from build123d import *

# Parameters (mm, degrees)
FILLET2_R = 2.1


with BuildPart() as part:
    # Sketch1 → Revolve1 (revolve)
    with BuildSketch(Plane(origin=(0, 0, 0), x_dir=(1, 0, 0), z_dir=(0, 1, 0)), mode=Mode.PRIVATE) as revolve1_sk:
        with BuildLine():
            Line((152.17858106, 53), (144.228415495, 53))
            ThreePointArc((144.228415495, 53), (136.67858106, 56), (129.128746624, 53))
            Line((129.128746624, 53), (121.17858106, 53))
            Line((121.17858106, 53), (121.17858106, 65))
            Line((121.17858106, 65), (152.17858106, 65))
            Line((152.17858106, 65), (152.17858106, 53))
        make_face()
    revolve(revolve1_sk.sketch.rotate(Axis((-165.426008969, 0, 0), (1, 0, 0)), 180), axis=Axis((-165.426008969, 0, 0), (1, 0, 0)))

    # Fillet2
    fillet2_edges = [part.edges().sort_by_distance(p)[0] for p in [
        (152.17858106, 0, -65),
        (121.17858106, 0, -65),
    ]]
    fillet(fillet2_edges, radius=FILLET2_R)


solid = part.part
Design review of the part built by this model. Coordinates are the model's own, in mm. Coordinates: 2 decimals unless noted, no trailing zeros. Order: outer loops, then holes, each group sorted by start corner. A loop starts at its lowest first (then second) coordinate and runs counter-clockwise, first axis right, second up.
Item 1: Take a section at C-C, the plane x = 139.5. Write out the cut boundary in (y, z), then the cut area to 3 significant figures.
Item 2: For pin 1 Ø8 at (x, y) = (130.5, 30.5) entering from -Z; pin 2 Ø8 at (x, y) = (141.5, -27) entering from -Z; pin 3 Ø1 at (x, y) = (147, -50.5) entering from -Z, all flat-tipped, find the tip position at first contact; note any pin that passes through.
Item 3: For line 1 (Y direction, x = 147.5, z = 0); line 2 (Z direction, x = 143.5, y = -1); line 3 (X direction, y = -44.5, z = -31.5), list the stretches that pass through material, from the lowest coordinate up.
Item 4: The part is to be moulded in two halves that separate along Z. For faces 1 (the cylindrical face through (136.87, -19.52, 62)), 2 (the cylindrical face through (148.15, -52.55, -6.9)), 3 (the flat face through (121.179, 42, 33)), say which applies: pulls with the +Z half, pulls with the -Z half, needs draft (parallel to the pull), parting line crosses it, or undercut.
Item 5: Take a section at A-A, the plane y = 0. Write out the cut boundary in (x, z), then the cut area to 3 significant figures.
The answers:
1. outline: circle Ø130 at (0, 0); hole circle Ø111.26 at (0, 0)
1. area: 3,550 mm2
2. pin 1: stops at z = -59.35
2. pin 2: stops at z = -60.79
2. pin 3: stops at z = -41.53
3. line 1: y = -65 to -53, 53 to 65
3. line 2: z = -64.99 to -53.62, 53.62 to 64.99
3. line 3: x = 121.18 to 131.17, 142.19 to 152.18
4. face 1: parting line crosses it
4. face 2: undercut
4. face 3: needs draft
5. outline: (121.18, -62.9) arc R2.1 ccw to (123.28, -65) - (150.08, -65) arc R2.1 ccw to (152.18, -62.9) - (152.18, -53) - (144.23, -53) arc R11 cw to (129.13, -53) - (121.18, -53) - close; (121.18, 53) - (129.13, 53) arc R11 cw to (144.23, 53) - (152.18, 53) - (152.18, 62.9) arc R2.1 ccw to (150.08, 65) - (123.28, 65) arc R2.1 ccw to (121.18, 62.9) - close
5. area: 678 mm2
